Can you work these out from the model? Positions are in its coordinate system, mm. Face numbers are marked on the shaded views. Coordinates: 2 decimals unless noted, no trailing zeros. Loops run counter-clockwise (first coordinate to the right, second up) from the corner with the lowest first, then second, coordinate; pieces in that order, holes last.
```python
from build123d import *

# Parameters (mm, degrees)
SKETCH1_W           = 117.602
SKETCH1_H           = 43.18
BOSS_EXTRUDE1_DEPTH = 12.319
SKETCH2_W           = 6.35
SKETCH2_H           = 12.7
CUT_EXTRUDE1_DEPTH  = 12.7
SKETCH3_W           = 30.280505476
SKETCH3_H           = 7.594186668
CUT_EXTRUDE2_DEPTH  = 12.7


with BuildPart() as part:
    # Sketch1 → Boss-Extrude1 (new, symmetric)
    with BuildSketch(Plane(origin=(0, 0, 0), x_dir=(1, 0, 0), z_dir=(0, 1, 0))):
        Rectangle(SKETCH1_W, SKETCH1_H)
    extrude(amount=BOSS_EXTRUDE1_DEPTH, both=True)

    # Sketch2 → Cut-Extrude1 (cut)
    with BuildSketch(Plane(origin=(0, 12.319, 0), x_dir=(1, 0, 0), z_dir=(0, 1, 0))):
        with Locations((45.466, -7.62)):
            Rectangle(SKETCH2_W, SKETCH2_H)
        with Locations((31.496, -7.62)):
            Rectangle(SKETCH2_W, SKETCH2_H)
        with Locations((17.526, -7.62)):
            Rectangle(SKETCH2_W, SKETCH2_H)
        with Locations((3.556, -7.62)):
            Rectangle(SKETCH2_W, SKETCH2_H)
        with Locations((-10.414, -7.62)):
            Rectangle(SKETCH2_W, SKETCH2_H)
        with Locations((-24.384, -7.62)):
            Rectangle(SKETCH2_W, SKETCH2_H)
        with Locations((-38.354, -7.62)):
            Rectangle(SKETCH2_W, SKETCH2_H)
    extrude(amount=-CUT_EXTRUDE1_DEPTH, mode=Mode.SUBTRACT)

    # Sketch3 → Cut-Extrude2 (cut)
    with BuildSketch(Plane.ZY.offset(58.801)):
        Rectangle(SKETCH3_W, SKETCH3_H)
    extrude(amount=-CUT_EXTRUDE2_DEPTH, mode=Mode.SUBTRACT)


solid = part.part
```
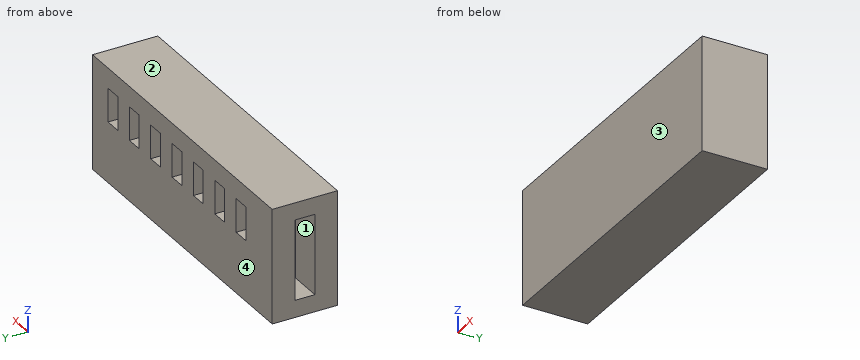
(1) I'm going to push a flat-ended pin straight in: pin 1 (3 mm diameter, centred on x = -24, z = 9.5, fed in from +Y). Where does the tip first touch, or does it pass through?
Check values:
pin 1: stops at y = -0.38
(2) I want a section at C-C on z = -11. Write out the boundary of the cut face in (x, y).
Check values:
outline: (-58.8, -12.32) - (58.8, -12.32) - (58.8, 12.32) - (-58.8, 12.32) - (-58.8, 3.8) - (-46.1, 3.8) - (-46.1, -3.8) - (-58.8, -3.8) - close
(3) If we mould it in two halves opening along Y, with no side actions, what happens to the marked faces 1, 2, 3 and 4? For each: released by +Y, released by -Y, zero draft, split by the parting line, or undercut.
Check values:
face 1: undercut
face 2: zero draft
face 3: released by -Y
face 4: released by +Y
(4) I want a section at A-A on y = 6. State how many separate pieces and enclosed holes the cut face has, then the cut area to 3 significant figures.
Check values:
separate pieces: 1
enclosed holes: 7
area: 4,510 mm2
(5) I want a section at B-B on x = -12. Write out the boundary of the cut face in (y, z).
Check values:
outline: (-12.32, -21.59) - (12.32, -21.59) - (12.32, 1.27) - (-0.38, 1.27) - (-0.38, 13.97) - (12.32, 13.97) - (12.32, 21.59) - (-12.32, 21.59) - close
(6) If I drill on probe 1 along Z at (x, y) = (-25.5, 6); probe 2 along Y at (x, z) = (1, 1.5); probe 3 along X at (y, z) = (-1.25, -4), over which ranges is the centre line in solid material (lowest first)?
Check values:
probe 1: z = -21.59 to 1.27, 13.97 to 21.59
probe 2: y = -12.32 to -0.38
probe 3: x = -46.1 to 58.8
